Verification items for the finished model (mm, model axes). Face numbers are marked on the shaded views. A direction names the side the tool comes from. Give positions to 0.01 mm unless a question says otherwise; leave off trailing zeros. Write each loop counter-clockwise with the first axis right and the second up, starting at its lowest first coordinate (ties: lowest second). Pieces come first, ordered by that corner, then holes. Notation, with made-up numbers: M 16.25,68.5 L 40.25,68.5 A11 cw 40.25,82.5 Z; hole C 0,40.5 d3. An arc over 180 degrees is marked long. Write item = value, one per line.
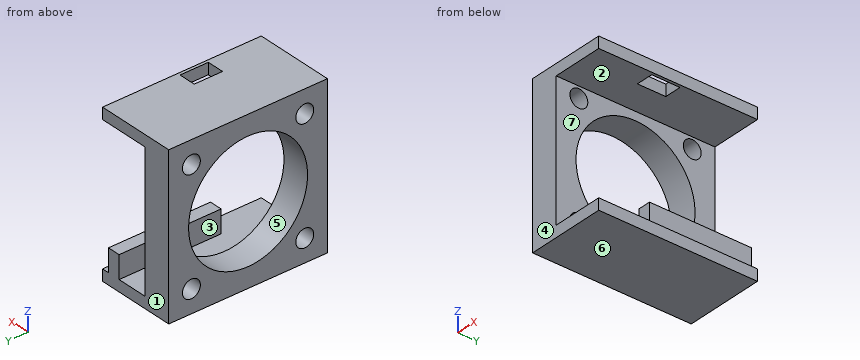
from build123d import *

# Parameters (mm, degrees)
SKETCH_W     = 28
SKETCH_H     = 28
SKETCH_R     = 1.58
SKETCH_R_2   = 10.5
PAD_DEPTH    = 5
SKETCH001_W  = 14
SKETCH001_H  = 28
PAD001_DEPTH = 2
SKETCH002_W  = 28
SKETCH002_H  = 14
PAD002_DEPTH = 2
SKETCH003_W  = 18
SKETCH003_H  = 4
PAD003_DEPTH = 2.25
SKETCH005_W  = 5
SKETCH005_H  = 3
POCKET_DEPTH = 5


with BuildPart() as part:
    # Sketch → Pad (new body)
    with BuildSketch(Plane.YZ):
        with Locations((14, 14)):
            Rectangle(SKETCH_W, SKETCH_H)
        with Locations((4, 24)):
            Circle(SKETCH_R, mode=Mode.SUBTRACT)
        with Locations((24, 24)):
            Circle(SKETCH_R, mode=Mode.SUBTRACT)
        with Locations((24, 4)):
            Circle(SKETCH_R, mode=Mode.SUBTRACT)
        with Locations((4, 4)):
            Circle(SKETCH_R, mode=Mode.SUBTRACT)
        with Locations((14, 14)):
            Circle(SKETCH_R_2, mode=Mode.SUBTRACT)
    extrude(amount=PAD_DEPTH)

    # Sketch001 → Pad001 (join)
    with BuildSketch(Plane.XY):
        with Locations((7, 14)):
            Rectangle(SKETCH001_W, SKETCH001_H)
    extrude(amount=PAD001_DEPTH)

    # Sketch002 (on DatumPlane) → Pad002 (join)
    with BuildSketch(Plane.YX.offset(-28)):
        with Locations((14, 7)):
            Rectangle(SKETCH002_W, SKETCH002_H)
    extrude(amount=PAD002_DEPTH)

    # Sketch003 (on DatumPlane) → Pad003 (join)
    with BuildSketch(Plane(origin=(10.5, -2, 0), x_dir=(0, 1, 0), z_dir=(1, 0, 0))):
        with Locations((21, 4)):
            Rectangle(SKETCH003_W, SKETCH003_H)
    extrude(amount=PAD003_DEPTH)

    # Sketch005 (on DatumPlane) → Pocket (cut)
    with BuildSketch(Plane.YX.offset(-28)):
        with Locations((12.25, 12)):
            Rectangle(SKETCH005_W, SKETCH005_H)
    extrude(amount=POCKET_DEPTH, mode=Mode.SUBTRACT)


solid = part.part
1) Draft check along Z on the marked faces 4, 5, 6 and 7. Enter one of: +Z half, -Z half, draft (parallel to the pull), parting line (faces both ways), or undercut.
From the geometry:
face_4 = draft
face_5 = undercut
face_6 = -Z half
face_7 = undercut
2) Cross-section at D-D on y = 8.75. Record the boundary of the cut face in (x, z).
From the geometry:
outline = M 0,0 L 14,0 L 14,2 L 5,2 L 5,4.91 L 0,4.91 Z; M 0,23.09 L 5,23.09 L 5,26 L 14,26 L 14,28 L 0,28 Z
3) Cross-section at B-B on z = 4. Record the boundary of the cut face in (x, y).
From the geometry:
outline = M 0,0 L 5,0 L 5,2.42 L 0,2.42 Z; M 0,5.58 L 5,5.58 L 5,10.8 L 0,10.8 Z; M 0,17.2 L 5,17.2 L 5,22.42 L 0,22.42 Z; M 0,25.58 L 5,25.58 L 5,28 L 0,28 Z; M 10.5,10 L 12.75,10 L 12.75,28 L 10.5,28 Z
4) Depth check by flat-ended pin: P1, Ø5, axis at x = 8.5, z = 7, coming from the -Y side; P2, Ø2, axis at y = 16, z = 3.5, coming from the +X side; P3, Ø2, axis at y = 20.5, z = 23, coming from the +X side. Enter the tip coordinate at first touch or a pass-through.
From the geometry:
P1 = 10
P2 = 12.75
P3 = 5
5) Cross-section at A-A on x = 6. Record the boundary of the cut face in (y, z), plus the area to 3 significant figures.
From the geometry:
outline = M 0,0 L 28,0 L 28,2 L 0,2 Z; M 0,26 L 28,26 L 28,28 L 0,28 Z
area = 112 mm^2
6) Tool access check on the marked faces 1, 2 and 3. Record the directions out of +Z, -Z, +X, -X, +Y, -Y that give a thin tool (end or side, any length) a straight path to the whole face; none if there is none.
From the geometry:
face_1 = +Z, -Z, +X, -X, +Y
face_2 = +X, +Y, -Y
face_3 = +Y, -Y
7) Cross-section at C-C on x = 11. Record the boundary of the cut face in (y, z), plus the area to 3 significant figures.
From the geometry:
outline = M 0,0 L 28,0 L 28,6 L 10,6 L 10,2 L 0,2 Z; M 0,26 L 9.75,26 L 9.75,28 L 0,28 Z; M 14.75,26 L 28,26 L 28,28 L 14.75,28 Z
area = 174 mm^2
8) Material ranges on probe 1 along Z at (x, y) = (1.5, 25); probe 2 along Z at (x, y) = (2.9, 14); probe 3 along Z at (x, y) = (10.5, 9.5), recorded low to high. Write a range as from..to.
From the geometry:
probe_1 = 0..2.78, 5.22..22.78, 25.22..28
probe_2 = 0..3.5, 24.5..28
probe_3 = 0..2, 26..28
